Verification items for the finished model (mm, model axes). Coordinates: 2 decimals unless noted, no trailing zeros. Write each loop counter-clockwise with the first axis right and the second up, starting at its lowest first coordinate (ties: lowest second). Pieces come first, ordered by that corner, then holes. Notation, with made-up numbers: (30.25, -22) -> (73.25, -22) arc R18 ccw to (73.25, -5) -> close; hole circle Ø1 at (-31.75, 6.25). An arc over 180 degrees is marked (long way). Use a Markdown table: item, result. Add a question column.
from build123d import *

# Parameters (mm, degrees)
SKETCH1_R                    = 76.2
SKETCH1_R_2                  = 15.875
PLATE_EXTRUDE_DEPTH          = 6.35
F_5_8_0_625_DIAMETER_HOLE1_D = 15.875
CIRPATTERN1_COUNT            = 6


with BuildPart() as part:
    # Sketch1 → Plate extrude (new body)
    with BuildSketch(Plane(origin=(0, 0, 0), x_dir=(1, 0, 0), z_dir=(0, 1, 0))):
        with Locations(Location((0, 0, 0), (0, 0, 270))):
            Circle(SKETCH1_R)
        with Locations(Location((0, 0, 0), (0, 0, 270))):
            Circle(SKETCH1_R_2, mode=Mode.SUBTRACT)
    extrude(amount=PLATE_EXTRUDE_DEPTH)

    # 5/8 (0.625) Diameter Hole1 (through all)
    with Locations(Plane(origin=(0, 6.35, 0), x_dir=(1, 0, 0), z_dir=(0, 1, 0))):
        with Locations((-50.8, 0)):
            f_5_8_0_625_diameter_hole1 = Hole(F_5_8_0_625_DIAMETER_HOLE1_D / 2)

    # CirPattern1: 5/8 (0.625) Diameter Hole1 ×6 about axis
    cirpattern1_axis = Axis((0, 0, 0), (0, 1, 0))
    for i in range(1, CIRPATTERN1_COUNT):
        add(f_5_8_0_625_diameter_hole1.rotate(cirpattern1_axis, i * 360 / CIRPATTERN1_COUNT), mode=Mode.SUBTRACT)


solid = part.part
1) Cross-section at D-D on y = 2.25. Give the number of separate pieces and of enclosed holes in the cut face, then the cut area to 3 significant figures.
2) Cross-section at B-B on z = -2.5. Record the boundary of the cut face in (x, y), then the cut area to 3 significant figures.
3) Thickness scan on L1, parallel to X at y = 1.75, z = -37; L2, parallel to Z at x = -25.4, y = 1.5; L3, parallel to X at y = 0.75, z = 2. Record the ranges inside material, lowest first.
4) Release check for a two-part mould opening along Z. For faces 1 (the face through (-46.367, 3.131, -60.47)), 2 (the face through (1, 0, 16)), 3 (the face through (21.737, 3.131, 51.036)) record: released by +Z, released by -Z, zero draft, split by the parting line, or undercut.
5) Gauge pin test, flat ends, axial feed: pin 1 (1.5 mm diameter, centred on y = 2.5, z = 48.5, fed in from +X); pin 2 (3 mm diameter, centred on y = 3, z = -46.5, fed in from -X); pin 3 (1 mm diameter, centred on x = 10, y = 5, fed in from +Z). Record the tip position at first contact, or that the pin passes through.
6) Cross-section at A-A on x = 0. Record the boundary of the cut face in (y, z) (3 decimals), then the cut area to 3 significant figures.
7) Cross-section at C-C on x = -25.4. Record the boundary of the cut face in (y, z), then the cut area to 3 significant figures.
Returned:
| question | item | result |
|---|---|---|
| 1 | separate pieces | 1 |
| 1 | enclosed holes | 7 |
| 1 | area | 16,300 mm² |
| 2 | outline | (-76.16, 0) -> (-58.33, 0) -> (-58.33, 6.35) -> (-76.16, 6.35) -> close; (-43.27, 0) -> (-15.68, 0) -> (-15.68, 6.35) -> (-43.27, 6.35) -> close; (15.68, 0) -> (43.27, 0) -> (43.27, 6.35) -> (15.68, 6.35) -> close; (58.33, 0) -> (76.16, 0) -> (76.16, 6.35) -> (58.33, 6.35) -> close |
| 2 | area | 577 mm² |
| 3 | L1 | x = -66.61 to -29.15, -21.65 to 21.65, 29.15 to 66.61 |
| 3 | L2 | z = -71.84 to -51.93, -36.06 to 36.06, 51.93 to 71.84 |
| 3 | L3 | x = -76.17 to -58.48, -43.12 to -15.75, 15.75 to 43.12, 58.48 to 76.17 |
| 4 | face 1 | split by the parting line |
| 4 | face 2 | zero draft |
| 4 | face 3 | undercut |
| 5 | pin 1 | stops at x = 59.38 |
| 5 | pin 2 | stops at x = -61.49 |
| 5 | pin 3 | stops at z = 75.61 |
| 6 | outline | (0, -76.2) -> (6.35, -76.2) -> (6.35, -15.875) -> (0, -15.875) -> close; (0, 15.875) -> (6.35, 15.875) -> (6.35, 76.2) -> (0, 76.2) -> close |
| 6 | area | 766 mm² |
| 7 | outline | (0, -71.84) -> (6.35, -71.84) -> (6.35, -51.93) -> (0, -51.93) -> close; (0, -36.06) -> (6.35, -36.06) -> (6.35, 36.06) -> (0, 36.06) -> close; (0, 51.93) -> (6.35, 51.93) -> (6.35, 71.84) -> (0, 71.84) -> close |
| 7 | area | 711 mm² |
